from build123d import *

# Parameters (mm, degrees)
ESQUISSE1_R                                = 18
BOSS_EXTRU_1_DEPTH                         = 65.18
BOSS_EXTRU_3_DEPTH                         = 6
BOSS_EXTRU_3_DEPTH_BACK                    = 16
ESQUISSE2_R                                = 11.25
ESQUISSE3_R                                = 4.8
ENL_V_MAT_EXTRU_1_DEPTH                    = 13
ESQUISSE4_R                                = 14
ENL_V_MAT_EXTRU_2_DEPTH                    = 9
ESQUISSE5_R                                = 10
ENL_V_MAT_EXTRU_3_DEPTH                    = 68.353117384
BOSS_EXTRU_4_DEPTH                         = 4
ESQUISSE9_R                                = 2
ENL_V_MAT_EXTRU_4_DEPTH                    = 74.994881031
ESQUISSE11_R                               = 4
ENL_V_MAT_EXTRU_5_DEPTH                    = 3.5
ESQUISSE12_R                               = 2
ENL_V_MAT_EXTRU_6_DEPTH                    = 3.5
SYM_TRIE4_AT_THE_SECOND_PLANE_COPY_1_SKE_R = 4
SYM_TRIE4_AT_THE_SECOND_PLANE_COPY_1_DEPTH = 3.5
SYM_TRIE4_AT_THE_SECOND_PLANE_COPY_2_SKE_R = 2
SYM_TRIE4_AT_THE_SECOND_PLANE_COPY_2_DEPTH = 3.5
ESQUISSE13_R                               = 13.25
ENL_V_MAT_EXTRU_7_DEPTH                    = 75
ENL_V_MAT_EXTRU_8_DEPTH                    = 10


with BuildPart() as part:
    # Esquisse1 → Boss.-Extru.1 (new body)
    with BuildSketch(Plane(origin=(0, 0, 0), x_dir=(1, 0, 0), z_dir=(0, 1, 0))):
        with Locations(Location((0, 0, 0), (0, 0, 270))):
            Circle(ESQUISSE1_R)
    extrude(amount=BOSS_EXTRU_1_DEPTH)

    # Esquisse2 → Boss.-Extru.3 (add, two sides: drawn at the far end of the back side and taken through both)
    with BuildSketch(Plane(origin=(-16.5, 0, 0), x_dir=(0, 0, -1), z_dir=(1, 0, 0)).offset(-BOSS_EXTRU_3_DEPTH_BACK)):
        with Locations((0, 33.87)):
            Circle(ESQUISSE2_R)
    extrude(amount=BOSS_EXTRU_3_DEPTH + BOSS_EXTRU_3_DEPTH_BACK)

    # Esquisse3 → Enlèv. mat.-Extru.1 (cut)
    with BuildSketch(Plane.ZY.offset(32.5)):
        with Locations((0, 33.87)):
            Circle(ESQUISSE3_R)
    extrude(amount=-ENL_V_MAT_EXTRU_1_DEPTH, mode=Mode.SUBTRACT)

    # Esquisse4 → Enlèv. mat.-Extru.2 (cut)
    with BuildSketch(Plane(origin=(0, 65.18, 0), x_dir=(1, 0, 0), z_dir=(0, 1, 0))):
        with Locations(Location((0, 0, 0), (0, 0, 270))):
            Circle(ESQUISSE4_R)
    extrude(amount=-ENL_V_MAT_EXTRU_2_DEPTH, mode=Mode.SUBTRACT)

    # Esquisse5 → Enlèv. mat.-Extru.3 (cut, through all)
    with BuildSketch(Plane(origin=(0, 56.18, 0), x_dir=(1, 0, 0), z_dir=(0, 1, 0))):
        with Locations(Location((0, 0, 0), (0, 0, 270))):
            Circle(ESQUISSE5_R)
    extrude(amount=-ENL_V_MAT_EXTRU_3_DEPTH, mode=Mode.SUBTRACT)

    # Esquisse8 → Boss.-Extru.4 (add)
    with BuildSketch(Plane(origin=(0, 0, 0), x_dir=(1, 0, 0), z_dir=(0, 1, 0))):
        with BuildLine():
            Line((13.645248867, 11.739130435), (2.274208144, 24.956521739))
            ThreePointArc((2.274208144, 24.956521739), (0, 26), (-2.274208144, 24.956521739))
            Line((-2.274208144, 24.956521739), (-13.645248867, 11.739130435))
            ThreePointArc((-13.645248867, 11.739130435), (0, 18), (13.645248867, 11.739130435))
        make_face()
    boss_extru_4 = extrude(amount=BOSS_EXTRU_4_DEPTH)

    # Esquisse9 → Enlèv. mat.-Extru.4 (cut, through all)
    with BuildSketch(Plane(origin=(0, 4, 0), x_dir=(1, 0, 0), z_dir=(0, 1, 0))):
        with Locations(Location((0, 21, 0), (0, 0, 270))):
            Circle(ESQUISSE9_R)
    enl_v_mat_extru_4 = extrude(amount=-ENL_V_MAT_EXTRU_4_DEPTH, mode=Mode.SUBTRACT)

    # Symétrie3: Boss.-Extru.4, Enlèv. mat.-Extru.4 across plane
    add(boss_extru_4.mirror(Plane(origin=(0, 0, 0), x_dir=(0, 0, 1), z_dir=(1, 0, 0))))
    add(enl_v_mat_extru_4.mirror(Plane(origin=(0, 0, 0), x_dir=(0, 0, 1), z_dir=(1, 0, 0))), mode=Mode.SUBTRACT)

    # Symétrie3 at the second plane: Boss.-Extru.4, Enlèv. mat.-Extru.4 across plane
    add(boss_extru_4.mirror(Plane.XY))
    add(enl_v_mat_extru_4.mirror(Plane.XY), mode=Mode.SUBTRACT)

    # Esquisse11 → Enlèv. mat.-Extru.5 (cut)
    with BuildSketch(Plane(origin=(0, 45.12, 0), x_dir=(1, 0, 0), z_dir=(0, 1, 0))):
        with Locations(Location((-26, 0, 0), (0, 0, 270))):
            Circle(ESQUISSE11_R)
    enl_v_mat_extru_5 = extrude(amount=-ENL_V_MAT_EXTRU_5_DEPTH, mode=Mode.SUBTRACT)

    # Esquisse12 → Enlèv. mat.-Extru.6 (cut)
    with BuildSketch(Plane(origin=(0, 41.62, 0), x_dir=(1, 0, 0), z_dir=(0, 1, 0))):
        with Locations(Location((-26, 0, 0), (0, 0, 270))):
            Circle(ESQUISSE12_R)
    enl_v_mat_extru_6 = extrude(amount=-ENL_V_MAT_EXTRU_6_DEPTH, mode=Mode.SUBTRACT)

    # Symétrie4: Enlèv. mat.-Extru.5, Enlèv. mat.-Extru.6 across plane
    add(enl_v_mat_extru_5.mirror(Plane.XY), mode=Mode.SUBTRACT)
    add(enl_v_mat_extru_6.mirror(Plane.XY), mode=Mode.SUBTRACT)

    # Symétrie4 at the second plane: Enlèv. mat.-Extru.5, Enlèv. mat.-Extru.6 across plane
    add(enl_v_mat_extru_5.mirror(Plane.ZX.offset(33.87)), mode=Mode.SUBTRACT)
    add(enl_v_mat_extru_6.mirror(Plane.ZX.offset(33.87)), mode=Mode.SUBTRACT)

    # Symétrie4 at the second plane copy 1 ske → Symétrie4 at the second plane copy 1 (cut)
    with BuildSketch(Plane.XZ.offset(-22.62)):
        with Locations(Location((-26, 0, 0), (0, 0, 270))):
            Circle(SYM_TRIE4_AT_THE_SECOND_PLANE_COPY_1_SKE_R)
    extrude(amount=-SYM_TRIE4_AT_THE_SECOND_PLANE_COPY_1_DEPTH, mode=Mode.SUBTRACT)

    # Symétrie4 at the second plane copy 2 ske → Symétrie4 at the second plane copy 2 (cut)
    with BuildSketch(Plane.XZ.offset(-26.12)):
        with Locations(Location((-26, 0, 0), (0, 0, 270))):
            Circle(SYM_TRIE4_AT_THE_SECOND_PLANE_COPY_2_SKE_R)
    extrude(amount=-SYM_TRIE4_AT_THE_SECOND_PLANE_COPY_2_DEPTH, mode=Mode.SUBTRACT)

    # Esquisse13 → Enlèv. mat.-Extru.7 (cut)
    with BuildSketch(Plane.XZ):
        with Locations(Location((0, 0, 0), (0, 0, 270))):
            Circle(ESQUISSE13_R)
    extrude(amount=-ENL_V_MAT_EXTRU_7_DEPTH, mode=Mode.SUBTRACT)

    # Esquisse14 → Enlèv. mat.-Extru.8 (cut)
    with BuildSketch(Plane(origin=(0, 4, 0), x_dir=(1, 0, 0), z_dir=(0, 1, 0))):
        with BuildLine():
            ThreePointArc((-2.44381305, -17.833333333), (0, -17), (2.44381305, -17.833333333))
            ThreePointArc((2.44381305, -17.833333333), (0, -18), (-2.44381305, -17.833333333))
        make_face()
    enl_v_mat_extru_8 = extrude(amount=ENL_V_MAT_EXTRU_8_DEPTH, mode=Mode.SUBTRACT)

    # Symétrie5: Enlèv. mat.-Extru.8 across plane
    add(enl_v_mat_extru_8.mirror(Plane.XY), mode=Mode.SUBTRACT)


solid = part.part
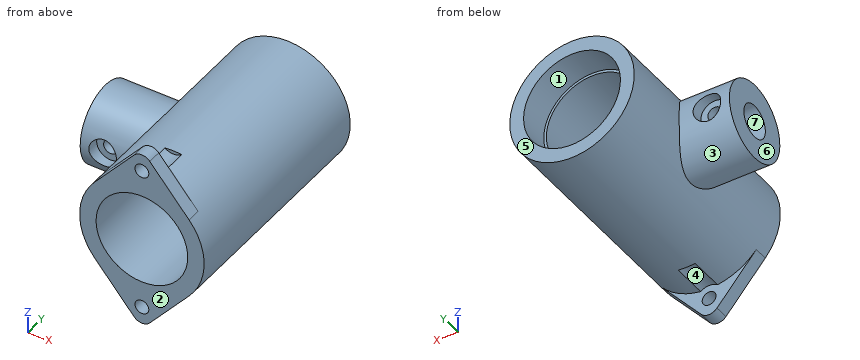
The model under review builds one solid part; all positions refer to its coordinate system, in mm. Face numbers are marked on the shaded views. A direction names the side the tool comes from. Coordinates: 2 decimals unless noted, no trailing zeros. Loops run counter-clockwise (first coordinate to the right, second up) from the corner with the lowest first, then second, coordinate; pieces in that order, holes last. Notation, with made-up numbers: M -29,32 L -22,32 A24 cw -22,46 Z; hole C -28.5,11.5 d2. An arc over 180 degrees is marked long. Put each result on its own line as item: value. Start each with the question number.
Q1. For the marked faces 1, 2, 3 and 4, list the 3-axis set-ups (+Z, -Z, +X, -X, +Y, -Y) from which the entire face can be reached by the end or side of a thin tool; tool diameter is ignored.
Q2. Add section B-B (x = 0). Write out the cut boundary in (y, z), and give its area (3 significant figures).
Q3. Wall thickness on line 1 (X direction, y = 40, z = 0); line 2 (X direction, y = 62, z = 0); line 3 (Z direction, x = 12, y = 20): over which ranges is each line inside the solid? List them lowest first.
Q4. Add section A-A (x = -26). Write out the cut boundary in (y, z), and give its area (3 significant figures).
Q5. The part is to be moulded in two halves that separate along Y. For the marked faces 5, 6 and 7, say which applies: +Y half, -Y half, draft (parallel to the pull), parting line (faces both ways), or undercut.
Q6. Add section D-D (z = -9.5). Write out the cut boundary in (x, y), and give its area (3 significant figures).
Q7. Add section C-C (y = 53.5). Write out the cut boundary in (x, z).
Q8. Clearance check with flat-ended pins moving along their axes: pin 1 (6 mm diameter, centred on x = -26.5, y = 45.5, fed in from +Z); pin 2 (6.5 mm diameter, centred on x = -26, z = 0, fed in from +Y); pin 3 (3.5 mm diameter, centred on x = 0, z = -21, fed in from -Y); pin 4 (2 mm diameter, centred on x = 6, y = 44, fed in from -Z). State where each tip first meets the part, or that it passes through.
Answers:
1. face 1: +Y
1. face 2: +Z, -Z, +X, -X, -Y
1. face 3: -X
1. face 4: -Z
2. outline: M 0,-26 L 4,-26 L 4,-23 L 0,-23 Z; M 0,-19 L 4,-19 L 4,-17 L 14,-17 L 14,-18 L 65.18,-18 L 65.18,-14 L 56.18,-14 L 56.18,-13.25 L 0,-13.25 Z; M 0,13.25 L 56.18,13.25 L 56.18,14 L 65.18,14 L 65.18,18 L 14,18 L 14,17 L 4,17 L 4,19 L 0,19 Z; M 0,23 L 4,23 L 4,26 L 0,26 Z
2. area: 618 mm^2
3. line 1: x = -32.5 to -28, -24 to -13.25, 13.25 to 18
3. line 2: x = -18 to -14, 14 to 18
3. line 3: z = -13.42 to -5.62, 5.62 to 13.42
4. outline: M 23.36,-4 A11.25 ccw 44.38,-4 L 41.62,-4 L 41.62,-2 L 38.23,-2 A4.8 cw 29.51,-2 L 26.12,-2 L 26.12,-4 Z; M 23.36,4 L 26.12,4 L 26.12,2 L 29.51,2 A4.8 cw 38.23,2 L 41.62,2 L 41.62,4 L 44.38,4 A11.25 ccw Z
4. area: 248 mm^2
5. face 5: +Y half
5. face 6: draft
5. face 7: undercut
6. outline: M -32.5,27.84 L -15.29,27.84 L -15.29,0 L -9.24,0 L -9.24,56.18 L -10.28,56.18 L -10.28,65.18 L -15.29,65.18 L -15.29,39.9 L -32.5,39.9 Z; M 9.24,0 L 15.29,0 L 15.29,65.18 L 10.28,65.18 L 10.28,56.18 L 9.24,56.18 Z
6. area: 978 mm^2
7. outline: C 0,0 d36; hole C 0,0 d26.5
8. pin 1: stops at z = 7.22
8. pin 2: stops at y = 41.62
8. pin 3: passes through
8. pin 4: stops at z = -17.29
